CAD build for the part. Positions are in the model's coordinates, mm. Face numbers are marked on the shaded views. Coordinates: 2 decimals unless noted, no trailing zeros. Order: outer loops, then holes, each group sorted by start corner. A loop starts at its lowest first (then second) coordinate and runs counter-clockwise, first axis right, second up. Notation, with made-up numbers: (34.25, -1) - (73.25, -1) arc R26 ccw to (73.25, 20) - close; hole circle Ø5 at (23.25, -12). An arc over 180 degrees is marked (long way). Return JSON: item names as keys, results as strings.
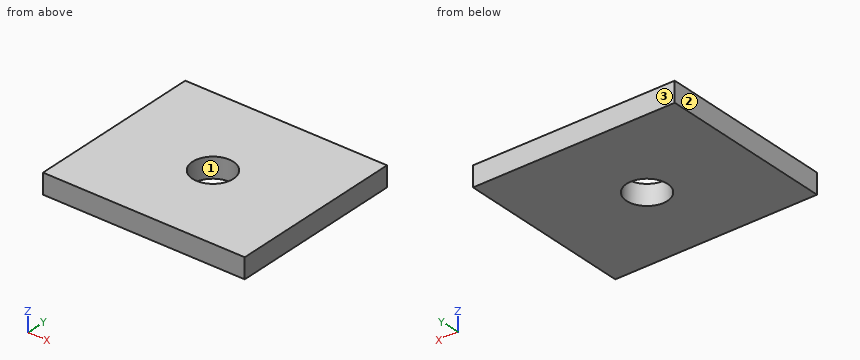
from build123d import *

# Parameters (mm, degrees)
SKETCH1_W                     = 40
SKETCH1_H                     = 35
PROFILE_DEPTH                 = 4
FASTENER_CLEARANCE_DEPTH      = 54.301031885
FASTENER_CLEARANCE_DEPTH_BACK = 54.301031885
SKETCH2_R                     = 4.05


with BuildPart() as part:
    # Sketch1 → Profile (new body)
    with BuildSketch(Plane.XY):
        with Locations((20, 17.5)):
            Rectangle(SKETCH1_W, SKETCH1_H)
    extrude(amount=PROFILE_DEPTH)

    # Sketch2 → Fastener_clearance (cut, two sides: drawn at the far end of the back side and taken through both)
    with BuildSketch(Plane.XY.offset(-FASTENER_CLEARANCE_DEPTH_BACK)):
        with Locations((20, 17)):
            Circle(SKETCH2_R)
    extrude(amount=FASTENER_CLEARANCE_DEPTH + FASTENER_CLEARANCE_DEPTH_BACK, mode=Mode.SUBTRACT)


solid = part.part
Item 1: Mould opens along Y. For the marked faces 1, 2 and 3 say: released by +Y, released by -Y, zero draft, split by the parting line, or undercut.
Findings below:
{"face 1": "undercut", "face 2": "zero draft", "face 3": "released by +Y"}
Item 2: Band-saw the part on A-A, the plane y = 17. List the corners of the cut face in (x, z), then the cut area to 3 significant figures.
Findings below:
{"outline": "(0, 0) - (15.95, 0) - (15.95, 4) - (0, 4) - close; (24.05, 0) - (40, 0) - (40, 4) - (24.05, 4) - close", "area": "128 mm²"}
Item 3: Band-saw the part on B-B, the plane x = 20. List the corners of the cut face in (y, z).
Findings below:
{"outline": "(0, 0) - (12.95, 0) - (12.95, 4) - (0, 4) - close; (21.05, 0) - (35, 0) - (35, 4) - (21.05, 4) - close"}
Item 4: Wall check: L1, parallel to Y at x = 20, z = 1; L2, parallel to X at y = 17, z = 1.7; L3, parallel to Y at x = 23, z = 2.65. Give the ranges that are in metal, low to high. Write a range as [from, to].
Findings below:
{"L1": "y = [0, 12.95], [21.05, 35]", "L2": "x = [0, 15.95], [24.05, 40]", "L3": "y = [0, 14.28], [19.72, 35]"}
Item 5: Band-saw the part on C-C, the plane z = 3.5. List the corners of the cut face in (x, y).
Findings below:
{"outline": "(0, 0) - (40, 0) - (40, 35) - (0, 35) - close; hole circle Ø8.1 at (20, 17)"}
